Check sheet for the modelled part. Datum: model origin and axes. Units: mm. Face numbers are marked on the shaded views. A direction names the side the tool comes from. Round coordinates to 2 decimals unless told otherwise and drop trailing zeros. Order: outer loops, then holes, each group sorted by start corner. A loop starts at its lowest first (then second) coordinate and runs counter-clockwise, first axis right, second up. Notation, with made-up numbers: (48.25, 13.5) -> (65.25, 13.5) arc R17 ccw to (65.25, 37.5) -> close; hole circle Ø1 at (-12.5, -5). An arc over 180 degrees is marked (long way). Use CSV: the item, a comma, the result in double quotes.
```python
from build123d import *

# Parameters (mm, degrees)
SKETCH_1_W          = 18.8
SKETCH_1_H          = 3.5
EXTRUDE_1_DEPTH     = 12.7
EXTRUDE_1_2_DEPTH   = 12.7
SKETCH_2_W          = 18.8
SKETCH_2_H          = 25.9
EXTRUDE_2_DEPTH     = 3.5
EXTRUDE_3_DEPTH     = 1.8
SKETCH_4_W          = 25.9
SKETCH_4_H          = 16.2
EXTRUDE_4_DEPTH     = 2
SKETCH_5_W          = 20.6
SKETCH_5_H          = 16.2
EXTRUDE_5_DEPTH     = 18.8
SKETCH_6_W          = 12.2
SKETCH_6_H          = 12.2
CUT_EXTRUDE_1_DEPTH = 18.8
FILLET_1_R          = 1.5
SKETCH_7_R          = 2.55
CUT_EXTRUDE_2_DEPTH = 18.8
SKETCH_9_R          = 0.75
CUT_EXTRUDE_3_DEPTH = 7


with BuildPart() as part:
    # Sketch 1 → Extrude 1 (new body)
    with BuildSketch(Plane(origin=(0, 0, 0), x_dir=(1, 0, 0), z_dir=(0, 1, 0))):
        with Locations((0, 11.2)):
            Rectangle(SKETCH_1_W, SKETCH_1_H)
    extrude(amount=EXTRUDE_1_DEPTH)



with BuildPart() as body_2:
    # Sketch 1 → Extrude 1 2 (new body)
    with BuildSketch(Plane(origin=(0, 0, 0), x_dir=(1, 0, 0), z_dir=(0, 1, 0))):
        with Locations((0, -11.2)):
            Rectangle(SKETCH_1_W, SKETCH_1_H)
    extrude(amount=EXTRUDE_1_2_DEPTH)


with BuildPart() as part_1:
    add(part.part)

    add(body_2.part)  # Extrude 2 merges body 2
    # Sketch 2 → Extrude 2 (add)
    with BuildSketch(Plane.XZ):
        Rectangle(SKETCH_2_W, SKETCH_2_H)
    extrude(amount=EXTRUDE_2_DEPTH)

    # Sketch 3 → Extrude 3 (add)
    with BuildSketch(Plane.ZY.offset(9.4)):
        Polygon((-12.95, 12.7), (-12.95, -3.5), (12.95, -3.5), (12.95, 12.7), (9.45, 12.7), (9.45, 0), (-9.45, 0), (-9.45, 12.7), align=None)
    extrude(amount=EXTRUDE_3_DEPTH)

    # Sketch 4 → Extrude 4 (add)
    with BuildSketch(Plane.ZY.offset(11.2)):
        with Locations((0, 4.6)):
            Rectangle(SKETCH_4_W, SKETCH_4_H)
    extrude(amount=EXTRUDE_4_DEPTH)

    # Sketch 5 → Extrude 5 (add)
    with BuildSketch(Plane.XY.offset(12.95)):
        with Locations((-0.9, 4.6)):
            Rectangle(SKETCH_5_W, SKETCH_5_H)
    extrude(amount=EXTRUDE_5_DEPTH)

    # Sketch 6 → Cut-Extrude 1 (cut)
    with BuildSketch(Plane.XY.offset(31.75)):
        with Locations((-0.9, 4.6)):
            Rectangle(SKETCH_6_W, SKETCH_6_H)
    extrude(amount=-CUT_EXTRUDE_1_DEPTH, mode=Mode.SUBTRACT)

    # Fillet 1
    fillet_1_edges = [part_1.edges().sort_by_distance(p)[0] for p in [
        (-11.2, 4.6, 12.95),
        (-0.9, -3.5, 31.75),
        (-0.9, 12.7, 31.75),
        (5.2, 10.7, 22.35),
        (5.2, -1.5, 22.35),
        (-7, -1.5, 22.35),
        (-7, 10.7, 22.35),
    ]]
    fillet(fillet_1_edges, radius=FILLET_1_R)

    # Sketch 7 → Cut-Extrude 2 (cut)
    with BuildSketch(Plane.XZ.offset(3.5)):
        with Locations(Location((-0.9, 22.35, 0), (0, 0, 90))):
            Circle(SKETCH_7_R)
    extrude(amount=-CUT_EXTRUDE_2_DEPTH, mode=Mode.SUBTRACT)

    # Sketch 9 → Cut-Extrude 3 (cut)
    with BuildSketch(Plane(origin=(0, 0, -12.95), x_dir=(-1, 0, 0), z_dir=(0, 0, -1))):
        with Locations((0.9, 5.35)):
            Circle(SKETCH_9_R)
        with Locations((6.9, 5.35)):
            Circle(SKETCH_9_R)
        with Locations((-5.1, 5.35)):
            Circle(SKETCH_9_R)
    extrude(amount=-CUT_EXTRUDE_3_DEPTH, mode=Mode.SUBTRACT)


solid = part_1.part
```
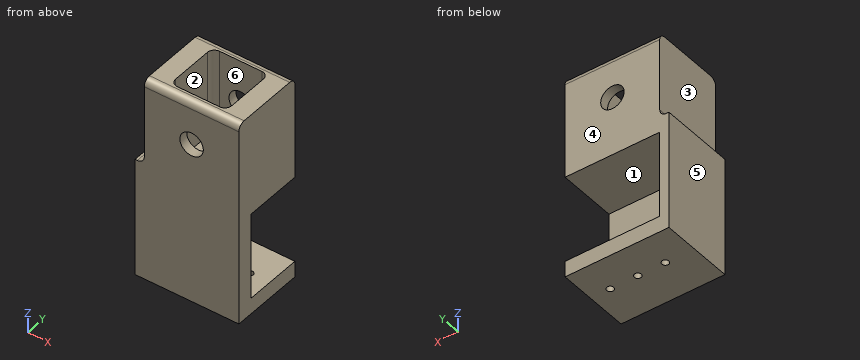
Q1. Sectioned sample at B-B, the plane z = 22.35. Enter the section's corners in (x, y).
Result sheet:
outline,"(-11.2, -3.5) -> (-3.45, -3.5) -> (-3.45, -1.5) -> (-5.5, -1.5) arc R1.5 cw to (-7, 0) -> (-7, 9.2) arc R1.5 cw to (-5.5, 10.7) -> (-3.45, 10.7) -> (-3.45, 12.7) -> (-11.2, 12.7) -> close; (1.65, -3.5) -> (9.4, -3.5) -> (9.4, 12.7) -> (1.65, 12.7) -> (1.65, 10.7) -> (3.7, 10.7) arc R1.5 cw to (5.2, 9.2) -> (5.2, 0) arc R1.5 cw to (3.7, -1.5) -> (1.65, -1.5) -> close"
Q2. Access from +Z, -Z, +X, -X, +Y, -Y to the whole of each face (thin tool, end or side, straight path). Record for the marked faces 1, 2 and 3.
Result sheet:
face 1,"+X, +Y"
face 2,"+Z"
face 3,"+Z, -X, +Y, -Y"
Q3. Sectioned sample at A-A, the plane x = -0.9. Enter the section's corners in (y, z).
Result sheet:
outline,"(-3.5, -12.95) -> (4.6, -12.95) -> (4.6, -9.45) -> (0, -9.45) -> (0, 9.45) -> (12.7, 9.45) -> (12.7, 19.8) -> (10.7, 19.8) -> (10.7, 12.95) -> (-1.5, 12.95) -> (-1.5, 19.8) -> (-3.5, 19.8) -> close; (-3.5, 24.9) -> (-1.5, 24.9) -> (-1.5, 31.75) -> (-2, 31.75) arc R1.5 ccw to (-3.5, 30.25) -> close; (6.1, -12.95) -> (12.7, -12.95) -> (12.7, -9.45) -> (6.1, -9.45) -> close; (10.7, 24.9) -> (12.7, 24.9) -> (12.7, 30.25) arc R1.5 ccw to (11.2, 31.75) -> (10.7, 31.75) -> close"
Q4. Go/stop test with flat-tipped pins: pin 1 (7.5 mm diameter, centred on y = 4, z = 17.5, fed in from -X); pin 2 (9.5 mm diameter, centred on x = 0.5, z = -4.5, fed in from +Y); pin 3 (1.4 mm diameter, centred on x = -0.9, y = 5.35, fed in from +Z). Record where each tip stops, or that it passes through.
Result sheet:
pin 1,"stops at x = -11.37"
pin 2,"stops at y = 0"
pin 3,"stops at z = 12.95"
Q5. Sectioned sample at D-D, the plane x = 2.5. Enter the section's corners in (y, z), then the cut area to 3 significant figures.
Result sheet:
outline,"(-3.5, -12.95) -> (12.7, -12.95) -> (12.7, -9.45) -> (0, -9.45) -> (0, 9.45) -> (12.7, 9.45) -> (12.7, 30.25) arc R1.5 ccw to (11.2, 31.75) -> (10.7, 31.75) -> (10.7, 12.95) -> (-1.5, 12.95) -> (-1.5, 31.75) -> (-2, 31.75) arc R1.5 ccw to (-3.5, 30.25) -> close"
area,"254 mm^2"
Q6. Sectioned sample at C-C, the plane y = 5.35. Enter the section's corners in (x, z), then the cut area to 3 significant figures.
Result sheet:
outline,"(-13.2, -12.95) -> (-7.65, -12.95) -> (-7.65, -9.45) -> (-11.2, -9.45) -> (-11.2, 9.45) -> (9.4, 9.45) -> (9.4, 31.75) -> (5.2, 31.75) -> (5.2, 12.95) -> (-7, 12.95) -> (-7, 31.75) -> (-11.2, 31.75) -> (-11.2, 14.45) arc R1.5 cw to (-12.7, 12.95) -> (-13.2, 12.95) -> close; (-6.15, -12.95) -> (-1.65, -12.95) -> (-1.65, -9.45) -> (-6.15, -9.45) -> close; (-0.15, -12.95) -> (4.35, -12.95) -> (4.35, -9.45) -> (-0.15, -9.45) -> close; (5.85, -12.95) -> (9.4, -12.95) -> (9.4, -9.45) -> (5.85, -9.45) -> close"
area,"339 mm^2"
Q7. Scan lines: L1, parallel to X at y = -2.5, z = 22.5; L2, parallel to Z at x = -3.5, y = 10.25; L3, parallel to Z at x = -9, y = 7.5. Record each from-to range of solid material in increasing order.
Result sheet:
L1,"x = -11.2 to -3.45, 1.65 to 9.4"
L2,"z = -12.95 to -9.45, 9.45 to 12.95"
L3,"z = -12.95 to -9.45, 9.45 to 31.75"
Q8. Mould release check, pull along X, two halves, no side actions. Record for the marked faces 4, 5 and 6: pulls with the +X half, pulls with the -X half, needs draft (parallel to the pull), parting line crosses it, or undercut.
Result sheet:
face 4,"needs draft"
face 5,"pulls with the -X half"
face 6,"undercut"
